Check sheet for the drawn part. Datum: minimum x, y, z corner. Units: mm. Give positions to 0.01 mm unless a question says otherwise; leave off trailing zeros. Loops run counter-clockwise (first coordinate to the right, second up) from the corner with the lowest first, then second, coordinate; pieces in that order, holes last.
1. Cross-section at B-B, the plane x = 105. Record the cut outline in (y, z), plus the area to 3 significant figures.
2. Cross-section at D-D, the plane y = 1.1. State how many separate pieces and enclosed holes the cut face has, plus the area to 3 significant figures.
3. Cross-section at C-C, the plane z = 66.5. Record the cut outline in (x, y).
4. Material ranges on L1, parallel to X at y = 0.45, z = 149; L2, parallel to Z at x = 110, y = 0.8; L3, parallel to X at y = 0.45, z = 72.5, recorded low to high.
5. Cross-section at A-A, the plane z = 155.5. Record the cut outline in (x, y).
6. Go/stop test with flat-tipped pins: pin 1 Ø12.5 at (x, z) = (75, 66.5) entering from +Y; pin 2 Ø1 at (y, z) = (2, 74) entering from +X; pin 3 Ø0.9 at (x, y) = (156.5, 2) entering from -Z; pin 4 Ø1.5 at (y, z) = (2, 90) entering from -X. Record where each tip stops, or that it passes through.
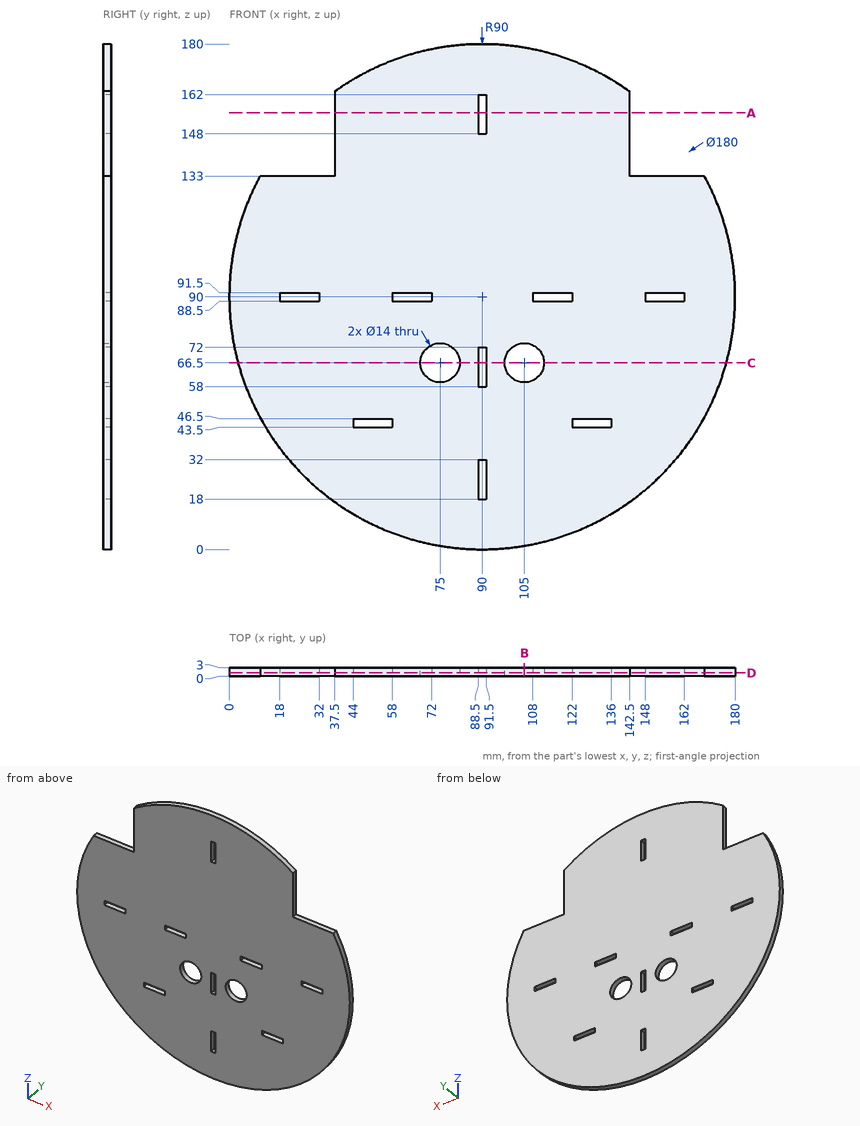
Result:
1. outline: (0, 1.26) - (3, 1.26) - (3, 59.5) - (0, 59.5) - close; (0, 73.5) - (3, 73.5) - (3, 178.74) - (0, 178.74) - close
1. area: 490 mm2
2. separate pieces: 1
2. enclosed holes: 11
2. area: 23,800 mm2
3. outline: (3.12, 0) - (68, 0) - (68, 3) - (3.12, 3) - close; (82, 0) - (88.5, 0) - (88.5, 3) - (82, 3) - close; (91.5, 0) - (98, 0) - (98, 3) - (91.5, 3) - close; (112, 0) - (176.88, 0) - (176.88, 3) - (112, 3) - close
4. L1: x = 37.5 to 88.5, 91.5 to 142.5
4. L2: z = 2.25 to 61.6, 71.4 to 88.5, 91.5 to 177.75
4. L3: x = 1.72 to 71.39, 78.61 to 101.39, 108.61 to 178.28
5. outline: (37.5, 0) - (88.5, 0) - (88.5, 3) - (37.5, 3) - close; (91.5, 0) - (142.5, 0) - (142.5, 3) - (91.5, 3) - close
6. pin 1: passes through
6. pin 2: stops at x = 178.66
6. pin 3: stops at z = 28.87
6. pin 4: stops at x = 0
